Build history of the part. All positions in model axes, mm. A direction names the side the tool comes from. Coordinates: 2 decimals unless noted, no trailing zeros. Write each loop counter-clockwise with the first axis right and the second up, starting at its lowest first coordinate (ties: lowest second). Pieces come first, ordered by that corner, then holes.
Solid Edge part; units mm, degrees
sketch "Sketch1" plane through (0, 0, 0) normal (0, -1, 0) x (1, 0, 0)
  arc A0 (-32, 16) -> (-36, 12) centre (-32, 12) ccw
  line L0 (-36, 12) -> (-36, -12)
  arc A1 (-36, -12) -> (-32, -16) centre (-32, -12) ccw
  line L1 (-32, -16) -> (32, -16)
  arc A2 (32, -16) -> (36, -12) centre (32, -12) ccw
  line L2 (36, -12) -> (36, 12)
  arc A3 (36, 12) -> (32, 16) centre (32, 12) ccw
  line L3 (32, 16) -> (-32, 16)
  arc A4 (-32, 20) -> (-40, 12) centre (-32, 12) ccw
  line L4 (-40, 12) -> (-40, -12)
  arc A5 (-40, -12) -> (-32, -20) centre (-32, -12) ccw
  line L5 (-32, -20) -> (32, -20)
  arc A6 (32, -20) -> (40, -12) centre (32, -12) ccw
  line L6 (40, -12) -> (40, 12)
  arc A7 (40, 12) -> (32, 20) centre (32, 12) ccw
  line L7 (32, 20) -> (-32, 20)
  dimension "D1" = 32
extrude "Protrusion1" add sketch "Sketch1" against normal blind 25.4
1. Probe line 1 along Z through (x, y) = (-11, 10.25); line 2 along X through (y, z) = (22.75, -0.5); line 3 along X through (y, z) = (8.5, -15). List the from-to ranges inside material, lowest first.
Computed values:
line 1: z = -20 to -16, 16 to 20
line 2: x = -40 to -36, 36 to 40
line 3: x = -39.42 to -34.65, 34.65 to 39.42
2. Mould opens along X. For faces 1 (the face through (0.2, 25.4, -16.2)), 2 (the face through (-34.797, 12.522, 14.859)), 3 (the face through (37.594, 12.522, -17.719)), 4 (the face through (-40, 13, 0)) say: +X half, -X half, draft (parallel to the pull), parting line (faces both ways), or undercut.
Computed values:
face 1: draft
face 2: undercut
face 3: +X half
face 4: -X half
3. Saw through at B-B on y = 17.5. List the corners of the cut face in (x, z).
Computed values:
outline: (-40, -12) arc R8 ccw to (-32, -20) - (32, -20) arc R8 ccw to (40, -12) - (40, 12) arc R8 ccw to (32, 20) - (-32, 20) arc R8 ccw to (-40, 12) - close; hole (-36, -12) arc R4 ccw to (-32, -16) - (32, -16) arc R4 ccw to (36, -12) - (36, 12) arc R4 ccw to (32, 16) - (-32, 16) arc R4 ccw to (-36, 12) - close
4. Saw through at A-A on x = 0.5. List the corners of the cut face in (y, z), plus the area to 3 significant figures.
Computed values:
outline: (0, -20) - (25.4, -20) - (25.4, -16) - (0, -16) - close; (0, 16) - (25.4, 16) - (25.4, 20) - (0, 20) - close
area: 203 mm2
5. Flat gauge pin, fed straight in: pin 1 (5 mm diameter, centred on y = 15, z = -16, fed in from +X). Where does the tip first touch, or does it go through?
Computed values:
pin 1: stops at x = 39.86
6. 3-axis set-ups, long thin cutter, end or side, ignore diameter. For faces 5 (the face through (37.719, 12.522, 17.594)), 6 (the face through (-34.859, 12.522, -14.797)): which of +Z, -Z, +X, -X, +Y, -Y reach the whole face in a straight line?
Computed values:
face 5: +Z, +X, +Y, -Y
face 6: +Y, -Y
7. Saw through at C-C on z = -6. List the corners of the cut face in (x, y).
Computed values:
outline: (-40, 0) - (-36, 0) - (-36, 25.4) - (-40, 25.4) - close; (36, 0) - (40, 0) - (40, 25.4) - (36, 25.4) - close
